from build123d import *

# Parameters (mm, degrees)
F0_W     = 254
F0_H     = 203.2
F1_DEPTH = 25.4
F2_W     = 12.7
F2_H     = 12.7
F3_DEPTH = 12.7
F4_R     = 1.27


with BuildPart() as f1:
    # F0 (on Top) → F1 (new body)
    with BuildSketch(Plane.XY):
        with Locations((127, 101.6)):
            Rectangle(F0_W, F0_H)
    extrude(amount=F1_DEPTH)

    # F2 (on face) → F3 (join)
    with BuildSketch(Plane.XY.offset(25.4)):
        with Locations((19.05, 184.15)):
            Rectangle(F2_W, F2_H)
    extrude(amount=F3_DEPTH)

    # F4
    f4_edges = [f1.edges().sort_by_distance(p)[0] for p in [
        (19.05, 177.8, 25.4),
        (25.4, 184.15, 25.4),
        (19.05, 190.5, 25.4),
        (12.7, 184.15, 25.4),
        (19.05, 190.5, 38.1),
        (12.7, 184.15, 38.1),
        (19.05, 177.8, 38.1),
        (25.4, 184.15, 38.1),
        (12.7, 177.8, 31.75),
        (25.4, 177.8, 31.75),
        (25.4, 190.5, 31.75),
        (12.7, 190.5, 31.75),
    ]]
    fillet(f4_edges, radius=F4_R)


solid = f1.part
For this review, take the finished solid that the model builds, in its own axes (mm). A direction names the side the tool comes from. Round coordinates to 2 decimals unless told otherwise and drop trailing zeros. Write each loop counter-clockwise with the first axis right and the second up, starting at its lowest first coordinate (ties: lowest second). Pieces come first, ordered by that corner, then holes. Notation, with made-up numbers: (54.25, 30.5) - (110.25, 30.5) arc R27 cw to (110.25, 53.5) - close; hole circle Ø1 at (9.25, -19). An arc over 180 degrees is marked (long way). Use a Markdown table: item, result.
Q1. We need section A-A (y = 183). Give the boundary of the cut face in (x, z), plus the area to 3 significant figures.
Derived:
| item | result |
|---|---|
| outline | (0, 0) - (254, 0) - (254, 25.4) - (26.67, 25.4) arc R1.27 cw to (25.4, 26.67) - (25.4, 36.83) arc R1.27 ccw to (24.13, 38.1) - (13.97, 38.1) arc R1.27 ccw to (12.7, 36.83) - (12.7, 26.67) arc R1.27 cw to (11.43, 25.4) - (0, 25.4) - close |
| area | 6,610 mm2 |
Q2. Clearance check with flat-ended pins moving along their axes: pin 1 (4 mm diameter, centred on y = 53, z = 21.5, fed in from -X); pin 2 (8 mm diameter, centred on x = 19, z = 33.5, fed in from +Y); pin 3 (12 mm diameter, centred on x = 162.5, y = 144.5, fed in from +Z); pin 4 (5 mm diameter, centred on x = 19.5, z = 32, fed in from -Y). State where each tip first meets the part, or that it passes through.
Derived:
| item | result |
|---|---|
| pin 1 | stops at x = 0 |
| pin 2 | stops at y = 190.5 |
| pin 3 | stops at z = 25.4 |
| pin 4 | stops at y = 177.8 |
Q3. Wall thickness on line 1 along Z through (x, y) = (74, 22.5): over which ranges is the line inside the solid? List them lowest first.
Derived:
| item | result |
|---|---|
| line 1 | z = 0 to 25.4 |
Q4. Machinability: for faces 1 (the flat face through (25.4, 184, 32)), 2 (the flat face through (19, 177.8, 32)), 3 (the flat face through (12.7, 184, 32)), which of the approach directions +Z, -Z, +X, -X, +Y, -Y give a long, thin tool a straight path to every point of the face, cutting with its end or side? Answer none if there is none.
Derived:
| item | result |
|---|---|
| face 1 | +Z, +X, +Y, -Y |
| face 2 | +Z, +X, -X, -Y |
| face 3 | +Z, -X, +Y, -Y |
Q5. We need section B-B (x = 120.5). Give the boundary of the cut face in (y, z), plus the area to 3 significant figures.
Derived:
| item | result |
|---|---|
| outline | (0, 0) - (203.2, 0) - (203.2, 25.4) - (0, 25.4) - close |
| area | 5,160 mm2 |
